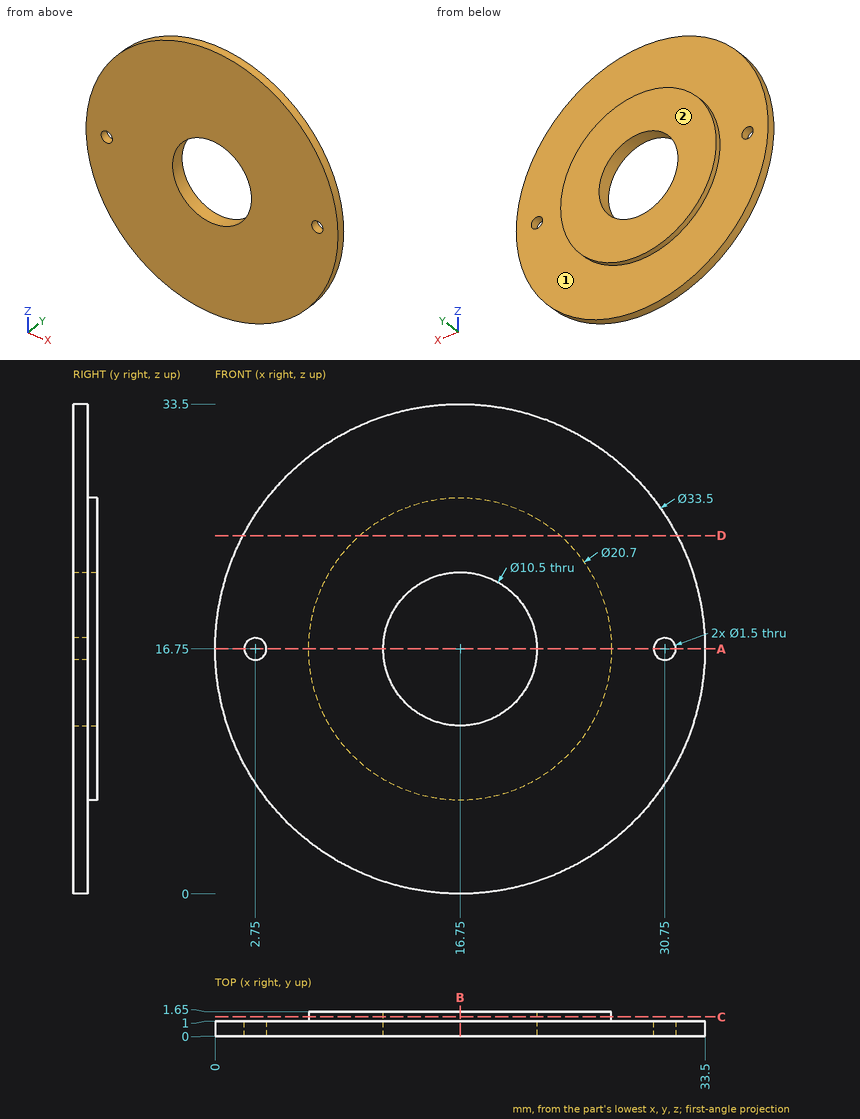
Answer from the drawing. Dimensions are ordinates in mm from the lowest x, y and z of the part. A direction names the side the tool comes from. Round coordinates to 2 decimals unless told otherwise and drop trailing zeros. Write each loop counter-clockwise with the first axis right and the second up, starting at its lowest first coordinate (ties: lowest second). Pieces come first, ordered by that corner, then holes. Notation, with made-up numbers: (-12, -1.75) - (14, -1.75) arc R12 ccw to (14, 19.25) - close; hole circle Ø1 at (-36, 23). An arc over 180 degrees is marked (long way). One line per item, written item: value.
Q1. Find section B-B (x = 16.75). Determine the outline of the cut face in (y, z), and give its area (3 significant figures).
The answers:
outline: (0, 0) - (1, 0) - (1, 6.4) - (1.65, 6.4) - (1.65, 11.5) - (0, 11.5) - close; (0, 22) - (1.65, 22) - (1.65, 27.1) - (1, 27.1) - (1, 33.5) - (0, 33.5) - close
area: 29.6 mm2
Q2. Which of the six approach directions +Z, -Z, +X, -X, +Y, -Y give full straight-line access (tool end or side, diameter ignored) to the marked faces 1 and 2?
The answers:
face 1: +Y
face 2: +Z, -Z, +X, -X, +Y
Q3. This flat-tipped pin is pushed along its axis until it touches: P1, Ø10, axis at x = 17, z = 18, coming from the +Y side. Where does it stop, or does it pass through?
The answers:
P1: stops at y = 1.65
Q4. Find section C-C (y = 1.3). Determine the outline of the cut face in (x, z), and give its area (3 significant figures).
The answers:
outline: circle Ø20.7 at (16.75, 16.75); hole circle Ø10.5 at (16.75, 16.75)
area: 250 mm2
Q5. Find section D-D (z = 24.5). Determine the outline of the cut face in (x, y).
The answers:
outline: (1.9, 0) - (31.6, 0) - (31.6, 1) - (23.61, 1) - (23.61, 1.65) - (9.89, 1.65) - (9.89, 1) - (1.9, 1) - close
Q6. Straight lines are drawn through the part: line 1 (X direction, y = 0.65, z = 16.75); line 2 (Z direction, x = 16.75, y = 1.2). For each, find the intervals that lie inside material, in ascending order. Write a range as from..to.
The answers:
line 1: x = 0..2, 3.5..11.5, 22..30, 31.5..33.5
line 2: z = 6.4..11.5, 22..27.1
Q7. Find section A-A (z = 16.75). Determine the outline of the cut face in (x, y), and give its area (3 significant figures).
The answers:
outline: (0, 0) - (2, 0) - (2, 1) - (0, 1) - close; (3.5, 0) - (11.5, 0) - (11.5, 1.65) - (6.4, 1.65) - (6.4, 1) - (3.5, 1) - close; (22, 0) - (30, 0) - (30, 1) - (27.1, 1) - (27.1, 1.65) - (22, 1.65) - close; (31.5, 0) - (33.5, 0) - (33.5, 1) - (31.5, 1) - close
area: 26.6 mm2
